Autodesk Inventor part; units mm, degrees
ref_plane "YZ Plane" through (0, 0, 0) normal (1, 0, 0) x (0, 1, 0)
ref_plane "XZ Plane" through (0, 0, 0) normal (0, 1, 0) x (-1, 0, 0)
ref_plane "XY Plane" through (0, 0, 0) normal (0, 0, 1) x (1, 0, 0)
sketch "Sketch1" plane through (0, 0, 0) normal (0, 0, 1) x (1, 0, 0)
  line L0 (0, 0) -> (25, 0)
  line L1 (25, 0) -> (25, 1.5)
  line L2 (25, 1.5) -> (0, 1.5)
  line L3 (0, 1.5) -> (0, 0)
  line L4 (0, 0) -> (-2.4, 0)
  line L5 (-2.4, 0) -> (-2.4, 2.75)
  line L6 (-2.4, 2.75) -> (0, 2.96)
  line L7 (0, 2.96) -> (0, 0)
  dimension "d0" = 3
  dimension "d3" = 25
  dimension "d46" = 85
  dimension "d47" = 2.4
  dimension "d49" = 5.5
revolve "Revolution1" add sketch "Sketch1" angle 360 about axis through (0, 0, 0) along (1, 0, 0)
thread "Thread1"
sketch "Sketch2" plane through (-2.4, 0, 0) normal (-1, 0, 0) x (0, 0, 1)
  circle A0 centre (0, 0) radius 1.4 construction
  circle A1 centre (0, 0) radius 0.98 construction
  line L0 (-0.8487, -0.49) -> (-1.4, 0)
  line L1 (0, 0) -> (-0.8487, -0.49)
  line L2 (0, 0) -> (-0.8487, 0.49)
  line L3 (-4.144, 0) -> (4.144, 0) construction
  line L4 (-1.4, 0) -> (-0.8487, 0.49)
  dimension "d21" = 2.8
  dimension "d19" = 60
  dimension "d20" = 30
  dimension "d26" = 1.96
extrude "Extrusion1" cut sketch "Sketch2" against normal blind 1.27
pattern_circular "Circular Pattern1" count 6 over 360 about axis through (-2.4, 0, 0) along (1, 0, 0) of "Extrusion1"
fillet "Fillet2" radius 0.3 6 edges at (-1.765, 1.2124, -0.7) (-1.765, 1.2124, 0.7) (-1.765, 0, 1.4) (-1.765, -1.2124, 0.7) (-1.765, -1.2124, -0.7) (-1.765, 0, -1.4)
fillet "Fillet3" radius 0.3 6 edges at (-1.765, 0.98, 0) (-1.765, 0.49, -0.8487) (-1.765, -0.49, -0.8487) (-1.765, -0.98, 0) (-1.765, -0.49, 0.8487) (-1.765, 0.49, 0.8487)
fillet "Fillet5" radius 0.1 1 edges at (0, -1.5, 0)
chamfer "Chamfer2" distance 0.3 angle 45 1 edges at (25, -1.5, 0)
equation "\"d6\" = b"
equation "\"d21\" = A_"
equation "\"d20\" = 0.5 * d19"
equation "\"d26\" = 0.7 * d21"
equation "\"d27\" = t"
equation "\"d32\" = v"
equation "\"d33\" = v"
equation "\"d35\" = r"
equation "\"d36\" = v"
equation "\"d0\" = d"
equation "\"d3\" = l_"
equation "\"d47\" = k"
equation "\"d49\" = dk"
equation "\"A_\" = 2.8"
equation "\"d\" = 3"
equation "\"dk\" = 5.5"
equation "\"k\" = 2.4"
equation "\"l_\" = 25"
equation "\"lg\" = 0"
equation "\"t\" = 1.27"
equation "\"w\" = 0.55"
equation "\"v\" = 0.3"
equation "\"r\" = 0.1"
equation "\"da\" = 2.6"
equation "\"ds_\" = d"
equation "\"ls\" = 0"
equation "\"b\" = l_ - lg"
equation "\"p\" = 0.5"
properties part number "Šroub s válcovou hlavou a šestiramennou drážkou ISO 14580 - M3x25-4.8" material "Ocel, měkká"
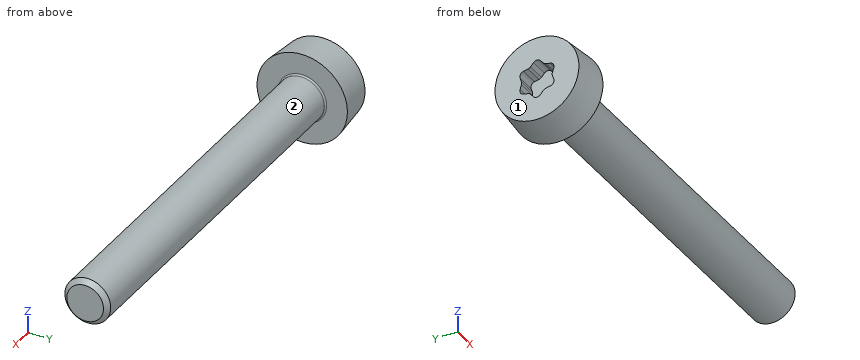
Work out the finished part from the listing and answer in its coordinate system (mm). Face numbers are marked on the shaded views. A direction names the side the tool comes from. Give positions to 0.01 mm unless a question says otherwise; leave off trailing zeros. Loops run counter-clockwise (first coordinate to the right, second up) from the corner with the lowest first, then second, coordinate; pieces in that order, holes last. Notation, with made-up numbers: (86.5, -13) -> (134.5, -13) arc R17 ccw to (134.5, 3) -> close; hole circle Ø8 at (-10, -23). An arc over 180 degrees is marked (long way). One line per question, with ' | ' between items. Start each with the question number.
1) For the marked faces 1 and 2, determine the directions among +Z, -Z, +X, -X, +Y, -Y from which every point of the face is accessible in a straight line to the end or side of a thin tool.
2) Straight lines are drawn through the part: L1, parallel to X at y = -1.35, z = 1.4; L2, parallel to X at y = -0.5, z = 0.2; L3, parallel to Y at x = 6.75, z = 0.1. For each, find the intervals that lie inside material, in ascending order.
3) Each of these flat-tipped pins is pushed along its axis until it touches: pin 1 (3 mm diameter, centred on y = -1, z = 1.5, fed in from +X); pin 2 (1.5 mm diameter, centred on x = 20.5, z = 0.5, fed in from -Y); pin 3 (3 mm diameter, centred on x = 17, y = 0, fed in from -Z); pin 4 (1.5 mm diameter, centred on x = 21, y = -2, fed in from -Z). Where does it stop, or does it pass through?
4) Section A-A, the plane x = 1.25 is taken. Determine the outline of the cut face in (y, z), then the cut area to 3 significant figures.
Resolved:
1) face 1: +Z, -Z, -X, +Y, -Y | face 2: +X
2) L1: -2.4 to 0 | L2: -1.13 to 25 | L3: -1.5 to 1.5
3) pin 1: x = 25 | pin 2: y = -1.5 | pin 3: z = -1.5 | pin 4: z = -0.83
4) outline: circle Ø3 at (0, 0) | area: 7.07 mm2
